Could you check a few things on this model? Use its own coordinates, in mm. Round coordinates to 2 decimals unless told otherwise and drop trailing zeros. Order: outer loops, then holes, each group sorted by start corner. A loop starts at its lowest first (then second) coordinate and runs counter-clockwise, first axis right, second up. Notation, with made-up numbers: M 53,50.5 L 92,50.5 A23 cw 92,80.5 Z; hole C 67,-13.75 d2. An arc over 180 degrees is marked long. Write each question's results on one line, items separated by ' | '. Start each with the question number.
1. Please list where this line runs through material, in increasing order: L1, parallel to X at y = -114, z = -125.65.
2. I'm going to push a flat-ended pin straight in: pin 1 (1.8 mm diameter, centred on x = 69.76, y = -114.03, fed in from +Z). Where does the tip first touch, or does it pass through?
3. We'd pull the mould along Y, two halves only. Please class faces 1 (the cylindrical face through (70.208, -115.458, -125.879)), 2 (the flat face through (90.314, -124, -126)), 3 (the flat face through (75, -143.527, -126)), 4 (the flat face through (75, -105.819, -126)): released by +Y, released by -Y, zero draft, split by the parting line, or undercut.
4. Suppose I cut it at A-A on y = -114.5. Write out the boundary of the cut face in (x, z).
from build123d import *

# Parameters (mm, degrees)
CIRCLE_R           = 1.5
EXTRUSION002_DEPTH = 51.281793
RECTANGLE_W        = 29.556112
RECTANGLE_H        = 37.708242
EXTRUSION001_DEPTH = 1


with BuildPart() as extrusion002:
    # Circle (on Extrusion) → Extrusion002 (new body)
    with BuildSketch(Plane(origin=(69.75761, -114.027299, -125.386342), x_dir=(0, -1, 0), z_dir=(0, 0, 1))):
        Circle(CIRCLE_R)
    extrude(amount=-EXTRUSION002_DEPTH)


with BuildPart() as cut001:
    # Rectangle (on Cut) → Extrusion001 (new body)
    with BuildSketch(Plane(origin=(60.75761, -105.819057, -125.386342), x_dir=(1, 0, 0), z_dir=(0, 0, -1))):
        with Locations((14.778056, 18.854121)):
            Rectangle(RECTANGLE_W, RECTANGLE_H)
    extrude(amount=EXTRUSION001_DEPTH)

    # Cut001: cut Extrusion002
    add(extrusion002.part, mode=Mode.SUBTRACT)


solid = cut001.part
Filled sheet:
1) L1: x = 60.76 to 68.26, 71.26 to 90.31
2) pin 1: passes through
3) face 1: undercut | face 2: zero draft | face 3: released by -Y | face 4: released by +Y
4) outline: M 60.76,-126.39 L 68.33,-126.39 L 68.33,-125.39 L 60.76,-125.39 Z; M 71.18,-126.39 L 90.31,-126.39 L 90.31,-125.39 L 71.18,-125.39 Z
